Source: CAD feature listing. Evaluate the final solid. Frame: model axes, mm. A direction names the side the tool comes from. Give positions to 0.01 mm unless a question says otherwise; leave off trailing zeros. Order: outer loops, then holes, each group sorted by start corner. A loop starts at its lowest first (then second) coordinate and runs counter-clockwise, first axis right, second up. Notation, with made-up numbers: (10, 88) -> (56, 88) arc R23 cw to (56, 118) -> close; hole circle Ø6 at (-12, 62.5). An arc over 180 degrees is marked (long way). Answer in a Markdown table with one row per item.
```python
from build123d import *

# Parameters (mm, degrees)
SKETCH1_W           = 30
SKETCH1_H           = 10
BOSS_EXTRUDE1_DEPTH = 0.5
SKETCH2_W           = 30
SKETCH2_H           = 3
BOSS_EXTRUDE2_DEPTH = 6
SKETCH3_W           = 30
SKETCH3_H           = 0.6
BOSS_EXTRUDE3_DEPTH = 5
FILLET1_R           = 3
FILLET2_R           = 1


with BuildPart() as part:
    # Sketch1 → Boss-Extrude1 (new body)
    with BuildSketch(Plane(origin=(0, 0, 0), x_dir=(1, 0, 0), z_dir=(0, 1, 0))):
        Rectangle(SKETCH1_W, SKETCH1_H)
    extrude(amount=BOSS_EXTRUDE1_DEPTH)

    # Sketch2 → Boss-Extrude2 (add)
    with BuildSketch(Plane(origin=(0, 0.5, 0), x_dir=(1, 0, 0), z_dir=(0, 1, 0))):
        with Locations((0, -3.5)):
            Rectangle(SKETCH2_W, SKETCH2_H)
    extrude(amount=BOSS_EXTRUDE2_DEPTH)

    # Sketch3 → Boss-Extrude3 (add)
    with BuildSketch(Plane.XY.offset(5)):
        with Locations((0, 6.2)):
            Rectangle(SKETCH3_W, SKETCH3_H)
    extrude(amount=BOSS_EXTRUDE3_DEPTH)

    # Fillet1
    fillet1_edges = [part.edges().sort_by_distance(p)[0] for p in [
        (0, 0.5, 2),
        (0, 5.9, 5),
    ]]
    fillet(fillet1_edges, radius=FILLET1_R)

    # Fillet2
    # the kernel refuses this fillet: 1 mm, written as the material it takes off along each edge
    with BuildSketch(Plane(origin=(17.291287847, 5.9, 10), x_dir=(0, 0, -1), z_dir=(-1, 0, 0))) as fillet2_piece_1:
        with BuildLine():
            CenterArc((0.916515139, -1), FILLET2_R, 90, 66.421821522)
            Line((0, -0.6), (-0.018330303, -0.592))
            ThreePointArc((-0.018330303, -0.592), (-0.02, -0.3), (-0.02, 0))
            Line((-0.02, 0), (0, 0.02))
            Line((0, 0.02), (0.916515139, 0.02))
            Line((0.916515139, 0.02), (0.916515139, 0))
        make_face()
    extrude(amount=34.582575695, mode=Mode.SUBTRACT)


solid = part.part
```
(1) Access query for faces 1 (the flat face through (-0.2, 5.9, 8.5)), 2 (the flat face through (0, 5, 2)), 3 (the flat face through (0, 0, 0)). Directions: +Z, -Z, +X, -X, +Y, -Y. A direction counts if a zero-diameter tool reaches every point of the face in a straight line with its end or side. Return the directions, or none.
A:
| item | result |
|---|---|
| face 1 | +Z, +X, -X, -Y |
| face 2 | -Z, +X, -X, +Y |
| face 3 | +Z, -Z, +X, -X, -Y |
(2) First-contact query: pin 1 Ø2.5 at (x, y) = (-6.5, 4.5) entering from -Z; pin 2 Ø1 at (x, z) = (10, 1) entering from +Y; pin 3 Ø1.2 at (x, z) = (-5, 8.5) entering from -Y. Flat tips, straight axial feed; report the tip coordinate or a pass-through.
A:
| item | result |
|---|---|
| pin 1 | stops at z = 1.99 |
| pin 2 | stops at y = 1.84 |
| pin 3 | stops at y = 5.9 |
(3) Ray query, probe 1 along Y at (x, z) = (2, -3.5); probe 2 along Y at (x, z) = (3, 8.25); probe 3 along Z at (x, y) = (-9, 5.5). Return the intervals inside material, ascending.
A:
| item | result |
|---|---|
| probe 1 | y = 0 to 0.5 |
| probe 2 | y = 5.9 to 6.5 |
| probe 3 | z = 2 to 6.5 |
(4) Section query C-C (y = 2). Return the cut outline in (x, z).
A:
| item | result |
|---|---|
| outline | (-15, 1.6) -> (15, 1.6) -> (15, 5) -> (-15, 5) -> close |
(5) Section query A-A (x = 6.5). Return the cut outline in (y, z), plus the area to 3 significant figures.
A:
| item | result |
|---|---|
| outline | (0, -5) -> (0.5, -5) -> (0.5, -1) arc R3 cw to (3.5, 2) -> (6.5, 2) -> (6.5, 10) arc R1 ccw to (5.9, 9.08) -> (5.9, 8) arc R3 cw to (2.9, 5) -> (0, 5) -> close |
| area | 29.7 mm^2 |
(6) Section query B-B (z = -2.5). Return the cut outline in (x, y).
A:
| item | result |
|---|---|
| outline | (-15, 0) -> (15, 0) -> (15, 0.5) -> (-15, 0.5) -> close |
